Verification items for the finished model (mm, model axes). Give positions to 0.01 mm unless a question says otherwise; leave off trailing zeros. Loops run counter-clockwise (first coordinate to the right, second up) from the corner with the lowest first, then second, coordinate; pieces in that order, holes last. Notation, with made-up numbers: (74.25, -13.75) - (99.25, -13.75) arc R16 ccw to (99.25, 0.25) - close; hole circle Ø6 at (17, -13.5). An arc over 180 degrees is marked (long way). One line per item, written item: value. Start each with the question number.
1. Sectioned sample at C-C (y = -24). Record the cut outline in (x, z).
2. Scan lines: L1, parallel to X at y = -21.5, z = 1.95; L2, parallel to X at y = -26.5, z = 1.75; L3, parallel to Y at x = 2.5, z = 1.4. Record each from-to range of solid material in increasing order. Write a range as [from, to].
3. Gauge pin test, flat ends, axial feed: pin 1 (5 mm diameter, centred on x = -47.88, y = -3.35, fed in from -Z); pin 2 (1 mm diameter, centred on y = -18.5, z = 1, fed in from -X); pin 3 (1 mm diameter, centred on y = -5, z = 1.5, fed in from -X). Record the tip position at first contact, or that the pin passes through.
4. Sectioned sample at D-D (x = -34). Record the cut outline in (y, z), plus the area to 3 significant figures.
5. Sectioned sample at B-B (z = 1.15). Record the cut outline in (x, y), plus the area to 3 significant figures.
6. Sectioned sample at A-A (y = 0). Record the cut outline in (x, z).
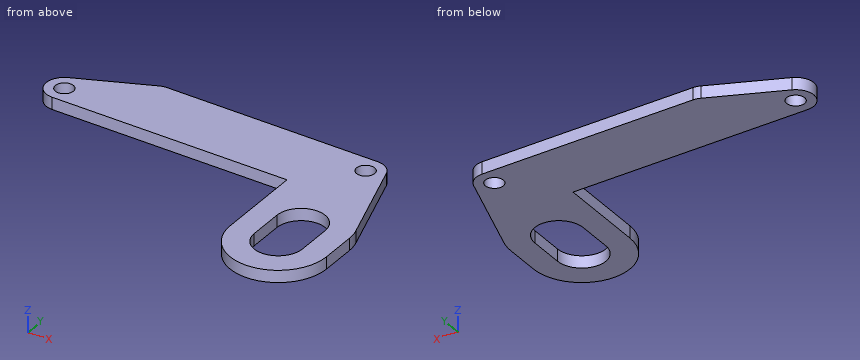
Autodesk Inventor part; units mm, degrees
ref_plane "YZ Plane" through (0, 0, 0) normal (1, 0, 0) x (0, 1, 0)
ref_plane "XZ Plane" through (0, 0, 0) normal (0, 1, 0) x (-1, 0, 0)
ref_plane "XY Plane" through (0, 0, 0) normal (0, 0, 1) x (1, 0, 0)
sketch "スケッチ1" plane through (0, 0, 0) normal (0, 0, 1) x (1, 0, 0)
  line L0 (0, 0) -> (0, -20) construction
  line L1 (0, -20) -> (-47.8831, -3.3483) construction
  line L2 (-47.8831, -3.3483) -> (0, 0) construction
  arc A0 (-49.007, -0.5668) -> (-48.0084, -6.3457) centre (-47.8831, -3.3483) ccw
  arc A1 (2.8673, 0.8824) -> (0.1253, 2.9974) centre (0, 0) ccw
  arc A2 (-8, -23) -> (8, -23) centre (0, -23) ccw
  arc A3 (4, -17) -> (-4, -17) centre (0, -17) ccw
  arc A4 (-4, -23) -> (4, -23) centre (0, -23) ccw
  line L3 (-4, -17) -> (-4, -23)
  line L4 (4, -17) -> (4, -23)
  line L5 (0, -23) -> (0, -17) construction
  line L6 (2.8673, 0.8824) -> (7.6462, -14.6471)
  line L7 (8, -17) -> (8, -23)
  arc A5 (8, -17) -> (7.6462, -14.6471) centre (0, -17) ccw
  line L8 (-49.007, -0.5668) -> (-37.007, 4.2821)
  line L9 (-35.7577, 4.498) -> (0.1253, 2.9974)
  arc A6 (-35.7577, 4.498) -> (-37.007, 4.2821) centre (-35.8831, 1.5006) ccw
  line L10 (-47.8831, -3.3483) -> (-35.8831, 1.5006) construction
  line L11 (-8, -23) -> (-8, -8.0188)
  line L12 (-8, -8.0188) -> (-48.0084, -6.3457)
  dimension "d0" = 20
  dimension "d2" = 48
  dimension "d3" = 3
  dimension "d13" = 6
  dimension "d14" = 4
  dimension "d15" = 8
  dimension "d17" = 3
  dimension "d18" = 4
  dimension "d20" = 12
  dimension "d21" = 86
extrude "押し出し1" add sketch "スケッチ1" along normal blind 2
hole "穴1" at (-47.8831, -3.3483, 0) at (0, 0, 0) direction (0, 0, 1) diameter 3 end through all
properties part number "COXA_YAW_SUPPORT-LINK_BACK"
Results are:
1. outline: (-7.94, 0) - (-3.87, 0) - (-3.87, 2) - (-7.94, 2) - close; (3.87, 0) - (7.94, 0) - (7.94, 2) - (3.87, 2) - close
2. L1: x = [-8, -4], [4, 8]
2. L2: x = [-7.19, -1.94], [1.94, 7.19]
2. L3: y = [-30.6, -26.12], [-13.88, 1.66]
3. pin 1: stops at z = 0
3. pin 2: stops at x = -8
3. pin 3: stops at x = -50.65
4. outline: (-6.93, 0) - (4.42, 0) - (4.42, 2) - (-6.93, 2) - close
4. area: 22.7 mm^2
5. outline: (-49.01, -0.57) arc R3 ccw to (-48.01, -6.35) - (-8, -8.02) - (-8, -23) arc R8 ccw to (8, -23) - (8, -17) arc R8 ccw to (7.65, -14.65) - (2.87, 0.88) arc R3 ccw to (0.13, 3) - (-35.76, 4.5) arc R3 ccw to (-37.01, 4.28) - close; hole circle Ø3 at (-47.88, -3.35); hole (-4, -23) arc R4 ccw to (4, -23) - (4, -17) arc R4 ccw to (-4, -17) - close; hole circle Ø3 at (0, 0)
5. area: 788 mm^2
6. outline: (-47.6, 0) - (-1.5, 0) - (-1.5, 2) - (-47.6, 2) - close; (1.5, 0) - (3.14, 0) - (3.14, 2) - (1.5, 2) - close
